Part model, mm, in its own coordinate system. A direction names the side the tool comes from. Round coordinates to 2 decimals unless told otherwise and drop trailing zeros. Loops run counter-clockwise (first coordinate to the right, second up) from the corner with the lowest first, then second, coordinate; pieces in that order, holes last.
1) Probe line 1 (Y direction, x = 0, z = 5.75) (3 decimals); line 2 (Y direction, x = 12.7, z = 8.75) (3 decimals); line 3 (Y direction, x = -1, z = 3.5). List the from-to ranges inside material, lowest first.
2) Band-saw the part on A-A, the plane y = -25.4. Write the cut outline in (x, z), then the cut area to 3 significant figures.
3) Band-saw the part on B-B, the plane x = 0. Write the cut outline in (y, z) (3 decimals).
4) Mould opens along Y. For faces 3 (the cylindrical face through (-1.915, -1.468, 6.261)), 4 (the flat face through (0, 5.461, 6)), 5 (the cylindrical face through (17.056, -49.655, 6.439)), 6 (the flat face through (4, -28, 12.7)) say: +Y half, -Y half, draft (parallel to the pull), parting line (faces both ways), or undercut.
5) Band-saw the part on C-C, the plane x = 12.7. Write the cut outline in (y, z) (3 decimals).
6) Band-saw the part on D-D, the plane z = 4.75. Write the cut outline in (x, y), then the cut area to 3 significant figures.
7) Drop flat-ended pins along their axis: P1, Ø2.5, axis at x = 12.7, y = -44.069, coming from the +Z side; P2, Ø6, axis at x = 13, z = 4.5, coming from the +Y side; P3, Ø6.5, axis at x = 0, y = 0, coming from the +Z side. Give the stop position or say it passes through.
8) 3-axis set-ups, long thin cutter, end or side, ignore diameter. For faces 1 (the flat face through (6, -50.419, 6)), 2 (the flat face through (5.08, -14, 6)): which of +Z, -Z, +X, -X, +Y, -Y reach the whole face in a straight line?
from build123d import *

# Parameters (mm, degrees)
SKETCH1_W           = 10.16
SKETCH1_H           = 38.1
SKETCH1_R           = 2.413
SKETCH1_R_2         = 2.286
BOSS_EXTRUDE1_DEPTH = 12.7
FILLET1_R           = 2.54


with BuildPart() as part:
    # Sketch1 → Boss-Extrude1 (new body)
    # profile 1 of 2: a face of its own
    with BuildSketch(Plane.XY):
        with Locations((0, -13.589)):
            Rectangle(SKETCH1_W, SKETCH1_H)
        with Locations((0, -25.4)):
            Circle(SKETCH1_R, mode=Mode.SUBTRACT)
        Circle(SKETCH1_R, mode=Mode.SUBTRACT)
    # profile 2 of 2: a face of its own
    with BuildSketch(Plane.XY):
        Polygon((5.08, -32.639), (-5.08, -32.639), (-5.08, -50.419), (17.78, -50.419), (17.78, -32.639), align=None)
        with Locations((0, -44.069)):
            Circle(SKETCH1_R_2, mode=Mode.SUBTRACT)
        with Locations((6.35, -37.719)):
            Circle(SKETCH1_R_2, mode=Mode.SUBTRACT)
        with Locations((12.7, -44.069)):
            Circle(SKETCH1_R_2, mode=Mode.SUBTRACT)
    extrude(amount=BOSS_EXTRUDE1_DEPTH)

    # Fillet1
    fillet1_edges = [part.edges().sort_by_distance(p)[0] for p in [
        (17.78, -50.419, 6.35),
        (-5.08, -50.419, 6.35),
        (-5.08, 5.461, 6.35),
        (5.08, 5.461, 6.35),
        (5.08, -32.639, 6.35),
        (17.78, -32.639, 6.35),
    ]]
    fillet(fillet1_edges, radius=FILLET1_R)


solid = part.part
Reported:
1. line 1: y = -50.419 to -46.355, -41.783 to -27.813, -22.987 to -2.413, 2.413 to 5.461
1. line 2: y = -50.419 to -46.355, -41.783 to -32.639
1. line 3: y = -50.42 to -46.12, -42.01 to -27.6, -23.2 to -2.2, 2.2 to 5.46
2. outline: (-5.08, 0) - (-2.41, 0) - (-2.41, 12.7) - (-5.08, 12.7) - close; (2.41, 0) - (5.08, 0) - (5.08, 12.7) - (2.41, 12.7) - close
2. area: 67.7 mm2
3. outline: (-50.419, 0) - (-46.355, 0) - (-46.355, 12.7) - (-50.419, 12.7) - close; (-41.783, 0) - (-27.813, 0) - (-27.813, 12.7) - (-41.783, 12.7) - close; (-22.987, 0) - (-2.413, 0) - (-2.413, 12.7) - (-22.987, 12.7) - close; (2.413, 0) - (5.461, 0) - (5.461, 12.7) - (2.413, 12.7) - close
4. face 3: undercut
4. face 4: +Y half
4. face 5: -Y half
4. face 6: draft
5. outline: (-50.419, 0) - (-46.355, 0) - (-46.355, 12.7) - (-50.419, 12.7) - close; (-41.783, 0) - (-32.639, 0) - (-32.639, 12.7) - (-41.783, 12.7) - close
6. outline: (-5.08, -47.88) arc R2.54 ccw to (-2.54, -50.42) - (15.24, -50.42) arc R2.54 ccw to (17.78, -47.88) - (17.78, -35.18) arc R2.54 ccw to (15.24, -32.64) - (7.62, -32.64) arc R2.54 cw to (5.08, -30.1) - (5.08, 2.92) arc R2.54 ccw to (2.54, 5.46) - (-2.54, 5.46) arc R2.54 ccw to (-5.08, 2.92) - close; hole circle Ø4.83 at (0, -25.4); hole circle Ø4.83 at (0, 0); hole circle Ø4.57 at (0, -44.07); hole circle Ø4.57 at (6.35, -37.72); hole circle Ø4.57 at (12.7, -44.07)
6. area: 702 mm2
7. P1: passes through
7. P2: stops at y = -32.64
7. P3: stops at z = 12.7
8. face 1: +Z, -Z, +X, -X, -Y
8. face 2: +Z, -Z, +X, +Y
